Geometry: final body of the model. Coordinates: model frame, mm. A direction names the side the tool comes from. Round coordinates to 2 decimals unless told otherwise and drop trailing zeros. Loops run counter-clockwise (first coordinate to the right, second up) from the corner with the lowest first, then second, coordinate; pieces in that order, holes last. Notation, with made-up numbers: M 36.5,45 L 69.5,45 A16 cw 69.5,70 Z; hole C 50.5,39 d10. An arc over 180 degrees is marked long. Answer as a JSON object with one key per item and string values.
```python
from build123d import *

# Parameters (mm, degrees)
F0_R      = 27.5
F0_R_2    = 26.5
F1_DEPTH  = 5
F2_R      = 27.5
F3_DEPTH  = 1
F5_DEPTH  = 25
F6_DEPTH  = 6
F8_D      = 9
F8_DEPTH  = 30
F8_TIP    = 2.7038727856
F9_DEPTH  = 25
F11_D     = 5
F11_DEPTH = 30
F11_TIP   = 1.5021515476
F12_R     = 30
F12_R_2   = 27.5
F13_DEPTH = 1


with BuildPart() as f1:
    # F0 (on Top) → F1 (new body)
    with BuildSketch(Plane.XY):
        Circle(F0_R)
        Circle(F0_R_2, mode=Mode.SUBTRACT)
    extrude(amount=F1_DEPTH)

    # F2 (on face) → F3 (join)
    with BuildSketch(Plane.XY.offset(5)):
        Circle(F2_R)
    extrude(amount=F3_DEPTH)

    # F4 (on Right) → F5 (join)
    with BuildSketch(Plane.YZ):
        Polygon((-8.5, 6), (0, 6), (8.5, 6), (-8.5, 16), align=None)
    extrude(amount=-F5_DEPTH)

    # F6 (cut): a face of the model
    f6_faces = [f1.faces().sort_by_distance(p)[0] for p in [
        (0, -2.8333333333, 9.3333333333),
    ]]
    extrude(f6_faces, amount=-F6_DEPTH, mode=Mode.SUBTRACT)

    # F8
    with Locations(Plane(origin=(0, 4.8071979434, 8.1722365039), x_dir=(1, 0, 0), z_dir=(0, 0.5070201266, 0.8619342152))):
        with Locations((-15.5, -5.5772213922)):
            Hole(F8_D / 2, depth=F8_DEPTH)
            with Locations((0, 0, -(F8_DEPTH + F8_TIP / 2))):  # 118° drill point
                Cone(0, F8_D / 2, F8_TIP, mode=Mode.SUBTRACT)

    # F9 (cut): a face of the model
    f9_faces = [f1.faces().sort_by_distance(p)[0] for p in [
        (-25, -2.8333333333, 9.3333333333),
    ]]
    extrude(f9_faces, amount=-F9_DEPTH, mode=Mode.SUBTRACT)

    # F11
    with Locations(Plane.XY.offset(6)):
        with Locations((0, 0)):
            Hole(F11_D / 2, depth=F11_DEPTH)
            with Locations((0, 0, -(F11_DEPTH + F11_TIP / 2))):  # 118° drill point
                Cone(0, F11_D / 2, F11_TIP, mode=Mode.SUBTRACT)

    # F12 (on face) → F13 (join)
    with BuildSketch(Plane.XY.offset(6)):
        Circle(F12_R)
        Circle(F12_R_2, mode=Mode.SUBTRACT)
    extrude(amount=-F13_DEPTH)


solid = f1.part
```
1) Cut plane A-A on x = 0. Return the cut outline in (y, z).
Geometry results:
{"outline": "M -30,5 L -27.5,5 L -27.5,0 L -26.5,0 L -26.5,5 L -2.5,5 L -2.5,6 L -30,6 Z; M 2.5,5 L 26.5,5 L 26.5,0 L 27.5,0 L 27.5,5 L 30,5 L 30,6 L 2.5,6 Z"}
2) Cut plane C-C on z = 3. Return the cut outline in (x, y).
Geometry results:
{"outline": "C 0,0 d55; hole C 0,0 d53"}
3) Cut plane D-D on x = -6. Return the cut outline in (y, z), and give its area (3 significant figures).
Geometry results:
{"outline": "M -29.39,5 L -26.84,5 L -26.84,0 L -25.81,0 L -25.81,5 L 25.81,5 L 25.81,0 L 26.84,0 L 26.84,5 L 29.39,5 L 29.39,6 L -29.39,6 Z", "area": "69.0 mm2"}
4) Set-up query: faces 1 (the face through (-5.961, -26.846, 2.465)), 2 (the face through (0.54, -2.44, 5.49)). Return all of +Z, -Z, +X, -X, +Y, -Y with unobstructed straight access to the full face (end or side cutting, diameter ignored); none if empty.
Geometry results:
{"face 1": "-Z", "face 2": "+Z, -Z"}
5) Cut plane B-B on y = -18. Return the cut outline in (x, z).
Geometry results:
{"outline": "M -24,5 L -20.79,5 L -20.79,0 L -19.45,0 L -19.45,5 L 19.45,5 L 19.45,0 L 20.79,0 L 20.79,5 L 24,5 L 24,6 L -24,6 Z"}
6) First-contact query: pin 1 (1.5 mm diameter, centred on y = 17, z = 5, fed in from -X); pin 2 (4 mm diameter, centred on x = 0, y = 0, fed in from +Z); pin 3 (1.5 mm diameter, centred on y = 11.5, z = 4, fed in from +X); pin 4 (2 mm diameter, centred on y = -14, z = 2.5, fed in from +X). Flat tips, straight axial feed; report the tip coordinate or a pass-through.
Geometry results:
{"pin 1": "x = -25.22", "pin 2": "through", "pin 3": "x = 25.31", "pin 4": "x = 24.23"}
7) Pull-direction query (Y, two-part tool) for faces 3 (the face through (-11, -3.2, 5.5)), 4 (the face through (6, 0, 6)), 5 (the face through (-29.97, 1.32, 5.51)); classes: +Y half, -Y half, draft (parallel to the pull), parting line (faces both ways), or undercut.
Geometry results:
{"face 3": "undercut", "face 4": "draft", "face 5": "parting line"}
8) Line query: probe 1 along Y at (x, z) = (0, 5.3); probe 2 along Y at (x, z) = (0, 3.65); probe 3 along X at (y, z) = (1.5, 5.75). Output: solid intervals per line, ascending.
Geometry results:
{"probe 1": "-30 to -2.5, 2.5 to 30", "probe 2": "-27.5 to -26.5, 26.5 to 27.5", "probe 3": "-29.96 to -17.65, -13.35 to -2, 2 to 29.96"}
